```python
from build123d import *

# Parameters (mm, degrees)
BOSS_EXTRUDE1_DEPTH = 4.3


with BuildPart() as part:
    # Sketch2 → Boss-Extrude1 (new body)
    with BuildSketch(Plane.XY):
        with BuildLine():
            Line((-25, -286), (-7.6, -286))
            Line((-7.6, -286), (-7.6, -290.3))
            Line((-7.6, -290.3), (7.6, -290.3))
            Line((7.6, -290.3), (7.6, -286))
            Line((7.6, -286), (25, -286))
            Line((25, -286), (25, -146.7666))
            Line((25, -146.7666), (29.3, -146.7666))
            Line((29.3, -146.7666), (29.3, -76.5666))
            Line((29.3, -76.5666), (25, -76.5666))
            Line((25, -76.5666), (25, 44.5667))
            ThreePointArc((25, 44.5667), (2.372583002, 53.939283002), (-7, 76.5667))
            Line((-7, 76.5667), (-7, 146.7667))
            ThreePointArc((-7, 146.7667), (2.372583002, 169.394116998), (25, 178.7667))
            Line((25, 178.7667), (25, 286))
            Line((25, 286), (7.6, 286))
            Line((7.6, 286), (7.6, 290.3))
            Line((7.6, 290.3), (-7.6, 290.3))
            Line((-7.6, 290.3), (-7.6, 286))
            Line((-7.6, 286), (-25, 286))
            Line((-25, 286), (-25, 146.7667))
            Line((-25, 146.7667), (-29.3, 146.7667))
            Line((-29.3, 146.7667), (-29.3, 76.5667))
            Line((-29.3, 76.5667), (-25, 76.5667))
            Line((-25, 76.5667), (-25, -44.5666))
            ThreePointArc((-25, -44.5666), (-2.372583002, -53.939183002), (7, -76.5666))
            Line((7, -76.5666), (7, -146.7666))
            ThreePointArc((7, -146.7666), (-2.372583002, -169.394016998), (-25, -178.7666))
            Line((-25, -178.7666), (-25, -286))
        make_face()
    extrude(amount=BOSS_EXTRUDE1_DEPTH)


solid = part.part
```
The model under review builds one solid part; all positions refer to its coordinate system, in mm. A direction names the side the tool comes from. Round coordinates to 2 decimals unless told otherwise and drop trailing zeros. Write each loop counter-clockwise with the first axis right and the second up, starting at its lowest first coordinate (ties: lowest second). Pieces come first, ordered by that corner, then holes. Notation, with made-up numbers: (21.5, 36) - (55.5, 36) arc R34 cw to (55.5, 68) - close; hole circle Ø1 at (-17.75, 45.5). An arc over 180 degrees is marked (long way). Use one line per item in the form item = value.
Q1. Consider section D-D (x = 18). State the section outline as (y, z) points.
Answer key:
outline = (-286, 0) - (45.34, 0) - (45.34, 4.3) - (-286, 4.3) - close; (177.99, 0) - (286, 0) - (286, 4.3) - (177.99, 4.3) - close
Q2. Draft analysis for pull direction Y (two halves, no side actions). For faces 1 (the flat face through (0, 4, 0)), 2 (the cylindrical face through (-2.125, -169.144, 2.12)), state which applies: +Y half, -Y half, draft (parallel to the pull), parting line (faces both ways), or undercut.
Answer key:
face_1 = draft
face_2 = undercut
Q3. For line 1 (Y direction, x = 23.5, z = 0.4); line 2 (Y direction, x = -2.5, z = 0.6); line 3 (X direction, y = -135, z = 2.2), list the stretches that pass through material, from the lowest coordinate up. Write a range as [from, to].
Answer key:
line_1 = [-286, 44.6], [178.73, 286]
line_2 = [-290.3, -169.52], [-53.81, 60.2], [163.13, 290.3]
line_3 = [7, 29.3]
Q4. Consider section B-B (z = 1.9). State the section outline as (x, y) points.
Answer key:
outline = (-29.3, 76.57) - (-25, 76.57) - (-25, -44.57) arc R32 cw to (7, -76.57) - (7, -146.77) arc R32 cw to (-25, -178.77) - (-25, -286) - (-7.6, -286) - (-7.6, -290.3) - (7.6, -290.3) - (7.6, -286) - (25, -286) - (25, -146.77) - (29.3, -146.77) - (29.3, -76.57) - (25, -76.57) - (25, 44.57) arc R32 cw to (-7, 76.57) - (-7, 146.77) arc R32 cw to (25, 178.77) - (25, 286) - (7.6, 286) - (7.6, 290.3) - (-7.6, 290.3) - (-7.6, 286) - (-25, 286) - (-25, 146.77) - (-29.3, 146.77) - close
Q5. Insertion check: pin 1 Ø1 at (x, z) = (-13, 2) entering from +Y; pin 2 Ø1 at (x, z) = (10, 3.5) entering from -Y; pin 3 Ø1.3 at (y, z) = (-100, 2) entering from -X. Each pin has a flat end and moves straight along its axis. Give the tip position at first contact, or say it passes through.
Answer key:
pin_1 = 286
pin_2 = -286
pin_3 = 7
Q6. Tool access review of faces 3 (the cylindrical face through (-2.623, -53.692, 2.12)), 4 (the flat face through (0, 4, 4.3)), 5 (the cylindrical face through (2.125, 169.144, 2.12)): name each direction out of +Z, -Z, +X, -X, +Y, -Y from which nothing blocks a thin tool from reaching the whole face with its end or side.
Answer key:
face_3 = +Z, -Z, -X
face_4 = +Z, +X, -X, +Y, -Y
face_5 = +Z, -Z, +X
Q7. Consider section A-A (x = -15). State the section outline as (y, z) points.
Answer key:
outline = (-286, 0) - (-177.16, 0) - (-177.16, 4.3) - (-286, 4.3) - close; (-46.17, 0) - (286, 0) - (286, 4.3) - (-46.17, 4.3) - close
Q8. Consider section C-C (y = -210). State the section outline as (x, z) points.
Answer key:
outline = (-25, 0) - (25, 0) - (25, 4.3) - (-25, 4.3) - close
